from build123d import *

# Parameters (mm, degrees)
SKETCH1_R           = 12.065
BOSS_EXTRUDE1_DEPTH = 23.3045
SKETCH2_W           = 2.286
SKETCH2_H           = 3.175
FILLET2_R           = 0.762
FILLET3_R           = 0.762


with BuildPart() as part:
    # Sketch1 → Boss-Extrude1 (new, symmetric)
    with BuildSketch(Plane(origin=(0, 0, 0), x_dir=(0, 0, -1), z_dir=(1, 0, 0))):
        Circle(SKETCH1_R)
    extrude(amount=BOSS_EXTRUDE1_DEPTH, both=True)

    # Sketch2 → Revolve1 (revolve)
    with BuildSketch(Plane.XY, mode=Mode.PRIVATE) as revolve1_sk:
        with Locations((24.4475, 1.5875)):
            Rectangle(SKETCH2_W, SKETCH2_H)
    revolve(revolve1_sk.sketch.rotate(Axis((23.3045, 0, 0), (-1, 0, 0)), 90), axis=Axis((23.3045, 0, 0), (-1, 0, 0)))

    # Fillet2
    fillet2_edges = [part.edges().sort_by_distance(p)[0] for p in [
        (23.3045, 0, 3.175),
        (25.5905, 0, 3.175),
    ]]
    fillet(fillet2_edges, radius=FILLET2_R)

    # Fillet3
    fillet3_edges = [part.edges().sort_by_distance(p)[0] for p in [
        (-23.3045, 0, 12.065),
        (23.3045, 0, 12.065),
    ]]
    fillet(fillet3_edges, radius=FILLET3_R)


solid = part.part
Verification items for the finished model (mm, model axes). A direction names the side the tool comes from. Coordinates: 2 decimals unless noted, no trailing zeros. Order: outer loops, then holes, each group sorted by start corner. A loop starts at its lowest first (then second) coordinate and runs counter-clockwise, first axis right, second up.
Item 1: Depth check by flat-ended pin: pin 1 (3 mm diameter, centred on x = 7.5, y = -4.5, fed in from +Z); pin 2 (8 mm diameter, centred on y = -7.5, z = 3.5, fed in from +X); pin 3 (4 mm diameter, centred on x = 18.5, y = 3.5, fed in from -Z). Enter the tip coordinate at first touch or a pass-through.
Filled in:
pin 1: stops at z = 11.69
pin 2: stops at x = 23.3
pin 3: stops at z = -11.97
Item 2: Section check C-C, the plane x = 1. Enter the section's corners in (y, z) (3 decimals).
Filled in:
outline: circle Ø24.13 at (0, 0)
Item 3: Material ranges on L1, parallel to X at y = 0, z = -10.5; L2, parallel to Z at x = -3, y = 0.25; L3, parallel to Y at x = 16.5, z = -0.5, recorded low to high.
Filled in:
L1: x = -23.3 to 23.3
L2: z = -12.06 to 12.06
L3: y = -12.05 to 12.05
Item 4: Access from +Z, -Z, +X, -X, +Y, -Y to the whole of each face (thin tool, end or side, straight path). Record for faces 1 (the face through (0.32, 3.62, -11.51)), 2 (the face through (24.45, 1.93, 2.52)).
Filled in:
face 1: +X, -X
face 2: +X
Item 5: Section check A-A, the plane y = 0. Enter the section's corners in (x, z) (1 decimal).
Filled in:
outline: (-23.3, -11.3) arc R0.8 ccw to (-22.5, -12.1) - (22.5, -12.1) arc R0.8 ccw to (23.3, -11.3) - (23.3, -3.9) arc R0.8 cw to (24.1, -3.2) - (24.8, -3.2) arc R0.8 ccw to (25.6, -2.4) - (25.6, 2.4) arc R0.8 ccw to (24.8, 3.2) - (24.1, 3.2) arc R0.8 cw to (23.3, 3.9) - (23.3, 11.3) arc R0.8 ccw to (22.5, 12.1) - (-22.5, 12.1) arc R0.8 ccw to (-23.3, 11.3) - close
